from build123d import *

# Parameters (mm, degrees)
ESBO_O1_W                                            = 42
ESBO_O1_H                                            = 65
RESSALTO_EXTRUS_O1_DEPTH                             = 21
ESBO_O2_W                                            = 17
ESBO_O2_H                                            = 22.225
CORTE_EXTRUS_O1_DEPTH                                = 43
FURO_COM_FOLGA_DE_M31_D                              = 3.4544
FURO_COM_FOLGA_DE_M31_DEPTH                          = 21
FURO_COM_FOLGA_DE_M201_D                             = 22.225
FURO_COM_FOLGA_DE_M201_DEPTH                         = 21
REBAIXO_PARA_PARAFUSO_DE_M_QUINA_DE_CABE_D           = 3.2
REBAIXO_PARA_PARAFUSO_DE_M_QUINA_DE_CABE_DEPTH       = 21
REBAIXO_PARA_PARAFUSO_DE_M_QUINA_DE_CABE_CBORE_D     = 6
REBAIXO_PARA_PARAFUSO_DE_M_QUINA_DE_CABE_CBORE_DEPTH = 7.62
FURO1_D                                              = 8.334375
FURO1_DEPTH                                          = 8
ESBO_O11_R                                           = 11.1125
ESBO_O11_R_2                                         = 5.5
RESSALTO_EXTRUS_O2_DEPTH                             = 4
ESBO_O12_W                                           = 42
ESBO_O12_H                                           = 65
ESBO_O12_R                                           = 5.5
ESBO_O12_R_2                                         = 1.6
ESBO_O12_R_3                                         = 1.7272
ESBO_O12_R_4                                         = 1.728196919
RESSALTO_EXTRUS_O3_DEPTH                             = 12
ESBO_O14_R                                           = 5.5
RESSALTO_EXTRUS_O4_DEPTH                             = 4


with BuildPart() as part:
    # Esboço1 → Ressalto-extrusão1 (new body)
    with BuildSketch(Plane.XY.offset(21)):
        with Locations((21, 32.5)):
            Rectangle(ESBO_O1_W, ESBO_O1_H)
    extrude(amount=-RESSALTO_EXTRUS_O1_DEPTH)

    # Esboço2 → Corte-extrusão1 (cut, through all)
    with BuildSketch(Plane(origin=(42, 0, 0), x_dir=(0, 0, -1), z_dir=(1, 0, 0))):
        with Locations((-8.5, 32.5)):
            Rectangle(ESBO_O2_W, ESBO_O2_H)
    extrude(amount=-CORTE_EXTRUS_O1_DEPTH, mode=Mode.SUBTRACT)

    # Furo com folga de M31
    with Locations(Plane(origin=(0, 0, 0), x_dir=(-1, 0, 0), z_dir=(0, 0, -1))):
        with Locations((-30, 7), (-16.7, 7), (-16.7, 58), (-30, 58)):
            Hole(FURO_COM_FOLGA_DE_M31_D / 2, depth=FURO_COM_FOLGA_DE_M31_DEPTH)

    # Furo com folga de M201
    with Locations(Plane.XY.offset(21)):
        with Locations((21, 32.5)):
            Hole(FURO_COM_FOLGA_DE_M201_D / 2, depth=FURO_COM_FOLGA_DE_M201_DEPTH)

    # Rebaixo para parafuso de máquina de cabeça sextavada de M31
    with Locations(Plane(origin=(0, 0, 0), x_dir=(-1, 0, 0), z_dir=(0, 0, -1))):
        with Locations((-36.5, 17), (-5.5, 17), (-5.5, 48), (-36.5, 48)):
            CounterBoreHole(REBAIXO_PARA_PARAFUSO_DE_M_QUINA_DE_CABE_D / 2, REBAIXO_PARA_PARAFUSO_DE_M_QUINA_DE_CABE_CBORE_D / 2, REBAIXO_PARA_PARAFUSO_DE_M_QUINA_DE_CABE_CBORE_DEPTH, depth=REBAIXO_PARA_PARAFUSO_DE_M_QUINA_DE_CABE_DEPTH)

    # Furo1
    with Locations(Plane(origin=(42, 0, 0), x_dir=(0, 0, -1), z_dir=(1, 0, 0))):
        with Locations((-14, 7), (-14, 58)):
            Hole(FURO1_D / 2, depth=FURO1_DEPTH)

    # Esboço11 → Ressalto-extrusão2 (add)
    with BuildSketch(Plane.XY.offset(21)):
        with Locations((21, 32.5)):
            Circle(ESBO_O11_R)
        with Locations((21, 32.5)):
            Circle(ESBO_O11_R_2, mode=Mode.SUBTRACT)
    extrude(amount=-RESSALTO_EXTRUS_O2_DEPTH)

    # Esboço12 → Ressalto-extrusão3 (add)
    with BuildSketch(Plane.XY.offset(21)):
        with Locations((21, 32.5)):
            Rectangle(ESBO_O12_W, ESBO_O12_H)
        with Locations((21, 32.5)):
            Circle(ESBO_O12_R, mode=Mode.SUBTRACT)
        with Locations((5.5, 48)):
            Circle(ESBO_O12_R_2, mode=Mode.SUBTRACT)
        with Locations((16.7, 58)):
            Circle(ESBO_O12_R_3, mode=Mode.SUBTRACT)
        with Locations((30, 58)):
            Circle(ESBO_O12_R_3, mode=Mode.SUBTRACT)
        with Locations((36.5, 48)):
            Circle(ESBO_O12_R_2, mode=Mode.SUBTRACT)
        with Locations((36.5, 17)):
            Circle(ESBO_O12_R_2, mode=Mode.SUBTRACT)
        with Locations((5.5, 17)):
            Circle(ESBO_O12_R_2, mode=Mode.SUBTRACT)
        with Locations((16.7, 7)):
            Circle(ESBO_O12_R_3, mode=Mode.SUBTRACT)
        with Locations((30, 7)):
            Circle(ESBO_O12_R_4, mode=Mode.SUBTRACT)
    extrude(amount=RESSALTO_EXTRUS_O3_DEPTH)

    # Esboço14 → Ressalto-extrusão4 (add)
    with BuildSketch(Plane.XY.offset(33)):
        with Locations((21, 32.5)):
            Circle(ESBO_O14_R)
    extrude(amount=-RESSALTO_EXTRUS_O4_DEPTH)


solid = part.part
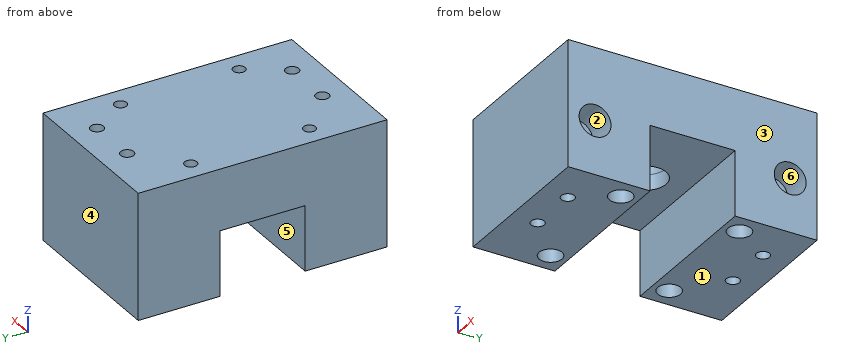
Check sheet for the modelled part. Datum: model origin and axes. Units: mm. Face numbers are marked on the shaded views. A direction names the side the tool comes from. Round coordinates to 2 decimals unless told otherwise and drop trailing zeros. Loops run counter-clockwise (first coordinate to the right, second up) from the corner with the lowest first, then second, coordinate; pieces in that order, holes last. Notation, with made-up numbers: M -35.5,14 L 17.5,14 A22 ccw 17.5,36 Z; hole C 23,21.25 d8. An arc over 180 degrees is marked long. One line per item, written item: value.
(1) Sectioned sample at A-A, the plane z = 14. Count the separate pieces of the cut face and the enclosed holes in it, then the cut area to 3 significant figures.
Computed values:
separate pieces: 2
enclosed holes: 8
area: 1,590 mm^2
(2) Sectioned sample at B-B, the plane y = 17. Record the cut outline in (x, z).
Computed values:
outline: M 0,0 L 2.5,0 L 2.5,7.62 L 3.9,7.62 L 3.9,33 L 0,33 Z; M 7.1,7.62 L 8.5,7.62 L 8.5,0 L 33.5,0 L 33.5,7.62 L 34.9,7.62 L 34.9,33 L 7.1,33 Z; M 38.1,7.62 L 39.5,7.62 L 39.5,0 L 42,0 L 42,33 L 38.1,33 Z
(3) Thickness scan on line 1 (Y direction, x = 36.5, z = 5.5); line 2 (Y direction, x = 30, z = 6); line 3 (Y direction, x = 11.5, z = 16). Record the ranges inside material, lowest first.
Computed values:
line 1: y = 0 to 14, 20 to 21.39, 43.61 to 45, 51 to 65
line 2: y = 0 to 5.27, 8.73 to 21.39, 43.61 to 56.27, 59.73 to 65
line 3: y = 0 to 21.39, 43.61 to 65
(4) Sectioned sample at D-D, the plane x = 36.5. Record the cut outline in (y, z).
Computed values:
outline: M 0,0 L 14,0 L 14,7.62 L 15.4,7.62 L 15.4,33 L 0,33 Z; M 18.6,7.62 L 20,7.62 L 20,0 L 21.39,0 L 21.39,17 L 43.61,17 L 43.61,0 L 45,0 L 45,7.62 L 46.4,7.62 L 46.4,33 L 18.6,33 Z; M 49.6,7.62 L 51,7.62 L 51,0 L 65,0 L 65,33 L 49.6,33 Z; hole C 7,14 d8.33; hole C 58,14 d8.33
(5) Depth check by flat-ended pin: pin 1 Ø5 at (x, y) = (5.5, 17) entering from +Z; pin 2 Ø5 at (x, y) = (5.5, 48) entering from -Z. Enter the tip coordinate at first touch or a pass-through.
Computed values:
pin 1: stops at z = 33
pin 2: stops at z = 7.62
(6) Access from +Z, -Z, +X, -X, +Y, -Y to the whole of each face (thin tool, end or side, straight path). Record for the marked faces 4, 5 and 6.
Computed values:
face 4: +Z, -Z, +X, -X, +Y
face 5: -Z, +X, -X
face 6: +X
(7) Release check for a two-part mould opening along Z. For the marked faces 1, 2 and 3 record: +Z half, -Z half, draft (parallel to the pull), parting line (faces both ways), or undercut.
Computed values:
face 1: -Z half
face 2: undercut
face 3: draft
